The listing builds one solid part. Answer for the finished solid, in the listing's coordinates (mm). Face numbers are marked on the shaded views. Give positions to 0.01 mm unless a question says otherwise; leave off trailing zeros. Loops run counter-clockwise (first coordinate to the right, second up) from the corner with the lowest first, then second, coordinate; pieces in that order, holes last. Notation, with made-up numbers: M 30,-13 L 55,-13 A25 cw 55,22 Z; hole C 75,29 d9. An arc over 180 degrees is marked long. Return JSON: item names as keys, results as strings.
from build123d import *

# Parameters (mm, degrees)
F0_W     = 112
F0_H     = 90.5
F1_DEPTH = 20
F3_DEPTH = 200
F4_W     = 103
F4_H     = 65.23
F5_DEPTH = 2.87
F6_W     = 109.5
F6_H     = 1.985677
F7_DEPTH = 3


with BuildPart() as f1:
    # F0 (on Front) → F1 (new body)
    with BuildSketch(Plane.XZ):
        Rectangle(F0_W, F0_H)
    extrude(amount=F1_DEPTH)

    # F2 (on face) → F3 (cut)
    with BuildSketch(Plane(origin=(-56, 0, 0), x_dir=(0, -1, 0), z_dir=(-1, 0, 0))):
        Polygon((5.75, -45.25), (0, 45.25), (0, -45.25), align=None)
    extrude(amount=-F3_DEPTH, mode=Mode.SUBTRACT)

    # F4 (on face) → F5 (cut)
    with BuildSketch(Plane.XZ.offset(20)):
        with Locations((0, -4.185)):
            Rectangle(F4_W, F4_H)
    extrude(amount=-F5_DEPTH, mode=Mode.SUBTRACT)

    # F6 (on face) → F7 (cut)
    with BuildSketch(Plane.XY.offset(45.25)):
        with Locations((0, -16.257161)):
            Rectangle(F6_W, F6_H)
    extrude(amount=-F7_DEPTH, mode=Mode.SUBTRACT)


solid = f1.part
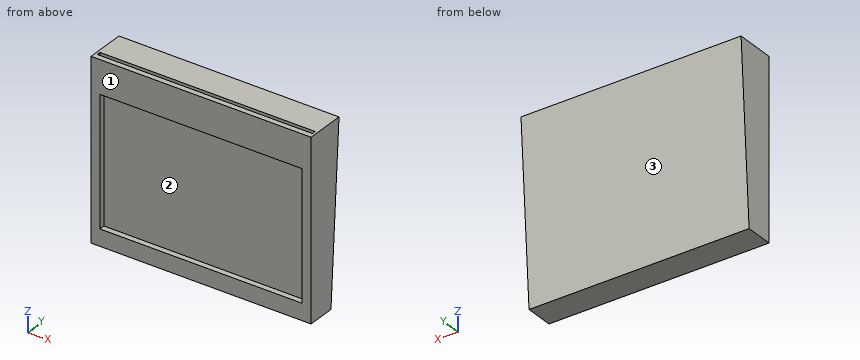
(1) Straight lines are drawn through the part: line 1 along X through (y, z) = (-19, -22.5); line 2 along Z through (x, y) = (43.5, -19); line 3 along Z through (x, y) = (25.5, -16.5). For each, find the intervals that lie inside material, in ascending order.
Values follow:
{"line 1": "-56 to -51.5, 51.5 to 56", "line 2": "-45.25 to -36.8, 28.43 to 45.25", "line 3": "-45.25 to 42.25"}
(2) Given pin 1 (2 mm diameter, centred on x = 7.5, y = -16.5, fed in from +Z); pin 2 (4 mm diameter, centred on x = -25, z = 21.5, fed in from +Y); pin 3 (1 mm diameter, centred on x = 7.5, z = 6.5, fed in from -Y); pin 4 (1 mm diameter, centred on x = -34.5, z = -26.5, fed in from +Y), each flat-ended and moving along its own axis, determine where each tip first touches the part or whether it passes through.
Values follow:
{"pin 1": "z = 45.25", "pin 2": "y = -1.38", "pin 3": "y = -17.13", "pin 4": "y = -4.53"}
(3) The part is cut by section A-A (x = 19). Determine the outline of the cut face in (y, z).
Values follow:
{"outline": "M -20,-45.25 L -5.75,-45.25 L 0,45.25 L -15.26,45.25 L -15.26,42.25 L -17.25,42.25 L -17.25,45.25 L -20,45.25 L -20,28.43 L -17.13,28.43 L -17.13,-36.8 L -20,-36.8 Z"}
(4) The part is cut by section D-D (z = -31). Determine the outline of the cut face in (x, y), and give its area (3 significant figures).
Values follow:
{"outline": "M -56,-20 L -51.5,-20 L -51.5,-17.13 L 51.5,-17.13 L 51.5,-20 L 56,-20 L 56,-4.84 L -56,-4.84 Z", "area": "1,400 mm²"}
(5) The part is cut by section B-B (z = 13). Determine the outline of the cut face in (x, y), and give its area (3 significant figures).
Values follow:
{"outline": "M -56,-20 L -51.5,-20 L -51.5,-17.13 L 51.5,-17.13 L 51.5,-20 L 56,-20 L 56,-2.05 L -56,-2.05 Z", "area": "1,710 mm²"}
(6) The part is cut by section C-C (y = -2.75). Determine the outline of the cut face in (x, z).
Values follow:
{"outline": "M -56,1.97 L 56,1.97 L 56,45.25 L -56,45.25 Z"}
(7) Determine the mould class of the marked faces 1, 2 and 3 for opening direction Z: released by +Z, released by -Z, zero draft, split by the parting line, or undercut.
Values follow:
{"face 1": "zero draft", "face 2": "undercut", "face 3": "released by -Z"}
